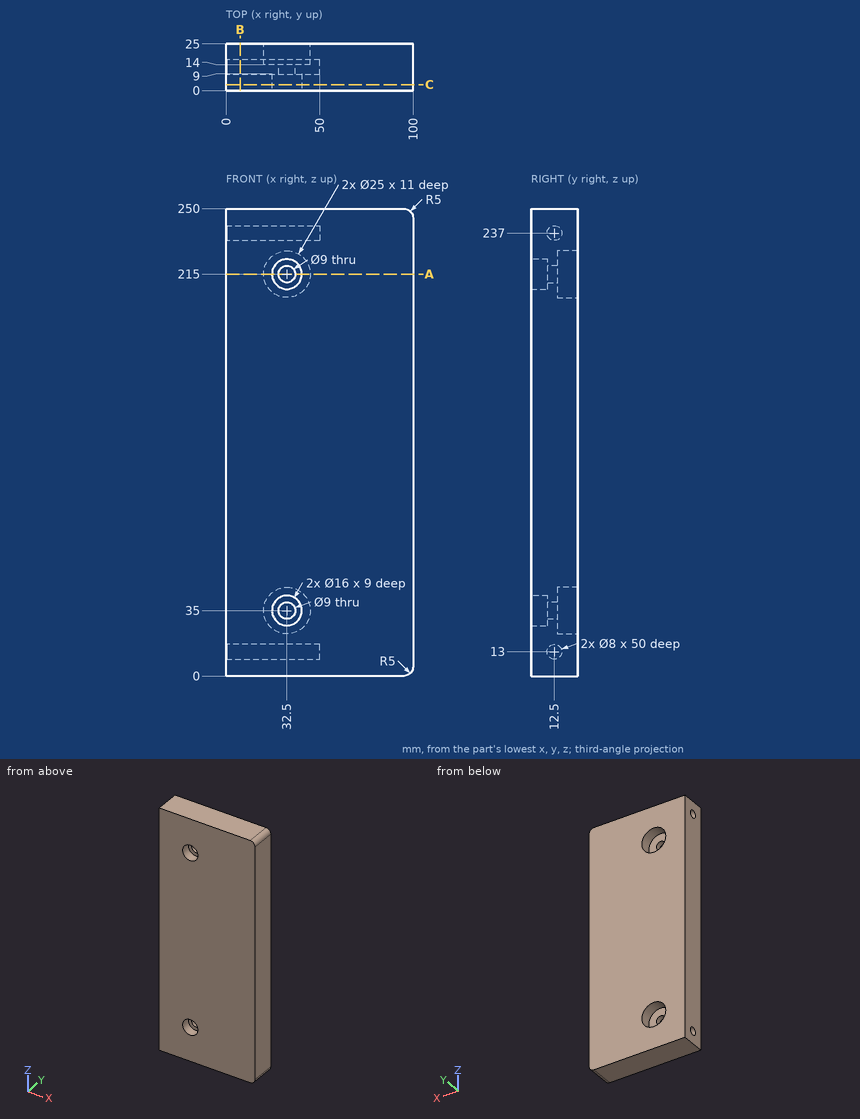
Here's the drawing with two shaded views (mm, measured from the low corner). I have some questions. Coordinates: 2 decimals unless noted, no trailing zeros. Loops run counter-clockwise (first coordinate to the right, second up) from the corner with the lowest first, then second, coordinate; pieces in that order, holes last. Notation, with made-up numbers: M 9.5,-18.75 L 66.5,-18.75 A20 ccw 66.5,8.25 Z; hole C -39,-6 d1. An arc over 180 degrees is marked long. Put each result on its own line as item: value. Start each with the question number.
(1) I need wall thicknesses on probe 1 along Y at (x, z) = (12, 237); probe 2 along X at (y, z) = (11.4, 35); probe 3 along Z at (x, y) = (27.5, 8) (3 decimals). Which ranges of each line are inside material? Lowest first, please.
(2) Imagine slicing it at C-C on y = 3.25. List the corners of the cut face in (x, z) for me.
(3) Imagine slicing it at B-B on x = 7.5. List the corners of the cut face in (y, z) for me, and give its area (3 significant figures).
(4) Will these pins go through, and if not, where does the flat tip stop? pin 1 Ø9.5 at (x, z) = (32.5, 35) entering from -Y; pin 2 Ø11.5 at (x, z) = (32.5, 215) entering from +Y; pin 3 Ø7 at (y, z) = (12.5, 13) entering from -X.
(5) Imagine slicing it at A-A on z = 215. List the corners of the cut face in (x, y) for me.
Worked answers:
1. probe 1: y = 0 to 8.5, 16.5 to 25
1. probe 2: x = 0 to 28, 37 to 100
1. probe 3: z = 0 to 28.755, 41.245 to 208.755, 221.245 to 250
2. outline: M 0,0 L 95,0 A5 ccw 100,5 L 100,245 A5 ccw 95,250 L 0,250 Z; hole C 32.5,35 d16; hole C 32.5,215 d16
3. outline: M 0,0 L 25,0 L 25,250 L 0,250 Z; hole C 12.5,13 d8; hole C 12.5,237 d8
3. area: 6,150 mm2
4. pin 1: stops at y = 9
4. pin 2: stops at y = 14
4. pin 3: stops at x = 50
5. outline: M 0,0 L 24.5,0 L 24.5,9 L 28,9 L 28,14 L 20,14 L 20,25 L 0,25 Z; M 37,9 L 40.5,9 L 40.5,0 L 100,0 L 100,25 L 45,25 L 45,14 L 37,14 Z
